The model under review builds one solid part; all positions refer to its coordinate system, in mm. A direction names the side the tool comes from. Give positions to 0.01 mm unless a question says otherwise; leave off trailing zeros. Order: outer loops, then holes, each group sorted by start corner. A loop starts at its lowest first (then second) coordinate and runs counter-clockwise, first axis right, second up. Notation, with made-up numbers: (22, 17.25) - (48, 17.25) arc R11 ccw to (48, 22.25) - close; hole circle Ø3 at (-19, 34.5). An arc over 180 degrees is marked (long way). Use CSV: the item, a comma, the result in double quotes. Start each with the question number.
```python
from build123d import *

# Parameters (mm, degrees)
SKETCH_4_W                  = 42
SKETCH_4_H                  = 42
EXTRUDE_2_DEPTH             = 26.3
CHAMFER_1_SIZE              = 4
FILLET_1_R                  = 2
SKETCH_5_R                  = 2
CUT_EXTRUDE_1_DEPTH         = 40.669761784
SKETCH_6_R                  = 4
SKETCH_6_R_2                = 3.5
EXTRUDE_3_DEPTH             = 1
EXTRUDE_START               = 1
SKETCH_7_R                  = 4
SKETCH_7_R_2                = 3.5
EXTRUDE_4_DEPTH             = 1
HOLE_WIZARD_M31_D           = 3.4
PATTERN_LINEAR_1_COUNT      = 2
PATTERN_LINEAR_1_PITCH      = 31
PATTERN_LINEAR_1_COUNT_DIR2 = 2
PATTERN_LINEAR_1_PITCH_DIR2 = 31


with BuildPart() as part:
    # Эскиз4 → Бобышка-Вытянуть2 (new body)
    with BuildSketch(Plane.XY):
        Rectangle(SKETCH_4_W, SKETCH_4_H)
    extrude(amount=EXTRUDE_2_DEPTH)

    # Фаска1
    chamfer_1_edges = [part.edges().sort_by_distance(p)[0] for p in [
        (21, -21, 13.15),
        (-21, -21, 13.15),
        (-21, 21, 13.15),
        (21, 21, 13.15),
    ]]
    chamfer(chamfer_1_edges, length=CHAMFER_1_SIZE)

    # Скругление1
    fillet_1_edges = [part.edges().sort_by_distance(p)[0] for p in [
        (0, -21, 0),
        (0, -21, 26.3),
        (21, 0, 0),
        (-21, 0, 0),
        (0, 21, 0),
        (-19, 19, 0),
        (19, 19, 0),
        (19, -19, 0),
        (-19, -19, 0),
        (-21, 0, 26.3),
        (21, 0, 26.3),
        (0, 21, 26.3),
        (-19, 19, 26.3),
        (19, 19, 26.3),
        (19, -19, 26.3),
        (-19, -19, 26.3),
    ]]
    fillet(fillet_1_edges, radius=FILLET_1_R)

    # Эскиз5 → Вырез-Вытянуть1 (cut, through all)
    with BuildSketch(Plane(origin=(0, 0, 0), x_dir=(-1, 0, 0), z_dir=(0, 0, -1))):
        Circle(SKETCH_5_R)
    extrude(amount=-CUT_EXTRUDE_1_DEPTH, mode=Mode.SUBTRACT)

    # Эскиз6 → Бобышка-Вытянуть3 (add)
    with BuildSketch(Plane(origin=(0, 0, 0), x_dir=(-1, 0, 0), z_dir=(0, 0, -1))):
        Circle(SKETCH_6_R)
        Circle(SKETCH_6_R_2, mode=Mode.SUBTRACT)
    extrude(amount=EXTRUDE_3_DEPTH)

    # Эскиз7 → Бобышка-Вытянуть4 (add)
    with BuildSketch(Plane.XY.offset(26.3).offset(EXTRUDE_START)):
        with Locations(Location((0, 0, 0), (0, 0, 180))):
            Circle(SKETCH_7_R)
        with Locations(Location((0, 0, 0), (0, 0, 180))):
            Circle(SKETCH_7_R_2, mode=Mode.SUBTRACT)
    extrude(amount=-EXTRUDE_4_DEPTH)

    # Отверстие с зазором M31 (through all)
    with Locations(Plane.XY.offset(26.3)):
        with Locations((-15.5, 15.5)):
            hole_wizard_m31 = Hole(HOLE_WIZARD_M31_D / 2)

    # Линейный массив1: Hole Wizard M31 2 × 2
    with Locations(*[(i * PATTERN_LINEAR_1_PITCH, -j * PATTERN_LINEAR_1_PITCH_DIR2, 0) for i in range(PATTERN_LINEAR_1_COUNT) for j in range(PATTERN_LINEAR_1_COUNT_DIR2) if (i, j) != (0, 0)]):
        add(hole_wizard_m31, mode=Mode.SUBTRACT)


solid = part.part
```
1. To check wall thickness, follow L1, parallel to Y at x = 0, z = 26.95; L2, parallel to Y at x = 15.5, z = 6; L3, parallel to X at y = 16, z = 20.25. State the ranges of each line that lie inside material, in increasing order. Write a range as [from, to].
2. Consider section C-C (z = 16). Give the boundary of the cut face in (x, y), and give its area (3 significant figures).
3. Consider section B-B (y = -15.5). Give the boundary of the cut face in (x, z), and give its area (3 significant figures).
4. Tool access review of faces 4 (the face through (19, 19, 13)), 5 (the face through (2, -2, 26.3)), 6 (the face through (2, -2, 0)): name each direction out of +Z, -Z, +X, -X, +Y, -Y from which nothing blocks a thin tool from reaching the whole face with its end or side.
5. Clearance check with flat-ended pins moving along their axes: pin 1 (19 mm diameter, centred on x = -3.5, y = -8.5, fed in from +Z); pin 2 (3 mm diameter, centred on x = -15.5, y = -15.5, fed in from -Z); pin 3 (5.5 mm diameter, centred on x = 0, y = 0, fed in from +Z); pin 4 (4.5 mm diameter, centred on x = 0, y = 0, fed in from -Z). State where each tip first meets the part, or that it passes through.
6. Consider section A-A (x = 0). Give the boundary of the cut face in (y, z), and give its area (3 significant figures).
7. Mouldability with a two-part tool opening along X and no side actions: class faces 1 (the face through (21, 0, 13)), 2 (the face through (-4.5, 0.3, 0)), 3 (the face through (-3.233, 1.341, 26.807)) as pulls with the +X half, pulls with the -X half, needs draft (parallel to the pull), parting line crosses it, or undercut.
Answers follow:
1,L1,"y = [-4, -3.5], [3.5, 4]"
1,L2,"y = [-21, -17.2], [-13.8, 13.8], [17.2, 21]"
1,L3,"x = [-21, -17.12], [-13.88, 13.88], [17.12, 21]"
2,outline,"(-21, -17) - (-17, -21) - (17, -21) - (21, -17) - (21, 17) - (17, 21) - (-17, 21) - (-21, 17) - close; hole circle Ø3.4 at (-15.5, -15.5); hole circle Ø3.4 at (-15.5, 15.5); hole circle Ø4 at (0, 0); hole circle Ø3.4 at (15.5, -15.5); hole circle Ø3.4 at (15.5, 15.5)"
2,area,"1,680 mm^2"
3,outline,"(-21, 2) arc R2 ccw to (-19, 0) - (-17.2, 0) - (-17.2, 26.3) - (-19, 26.3) arc R2 ccw to (-21, 24.3) - close; (-13.8, 0) - (13.8, 0) - (13.8, 26.3) - (-13.8, 26.3) - close; (17.2, 0) - (19, 0) arc R2 ccw to (21, 2) - (21, 24.3) arc R2 ccw to (19, 26.3) - (17.2, 26.3) - close"
3,area,"922 mm^2"
4,face 4,"+Z, -Z, +X, +Y"
4,face 5,"+Z"
4,face 6,"-Z"
5,pin 1,"stops at z = 27.3"
5,pin 2,"passes through"
5,pin 3,"stops at z = 26.3"
5,pin 4,"stops at z = 0"
6,outline,"(-21, 2) arc R2 ccw to (-19, 0) - (-4, 0) - (-4, -1) - (-3.5, -1) - (-3.5, 0) - (-2, 0) - (-2, 26.3) - (-3.5, 26.3) - (-3.5, 27.3) - (-4, 27.3) - (-4, 26.3) - (-19, 26.3) arc R2 ccw to (-21, 24.3) - close; (2, 0) - (3.5, 0) - (3.5, -1) - (4, -1) - (4, 0) - (19, 0) arc R2 ccw to (21, 2) - (21, 24.3) arc R2 ccw to (19, 26.3) - (4, 26.3) - (4, 27.3) - (3.5, 27.3) - (3.5, 26.3) - (2, 26.3) - close"
6,area,"998 mm^2"
7,face 1,"pulls with the +X half"
7,face 2,"needs draft"
7,face 3,"undercut"
